Geometry check sheet. Reference: drawing and pictorial views, mm from the part's lowest x, y, z. A direction names the side the tool comes from. Coordinates: 2 decimals unless noted, no trailing zeros. Write each loop counter-clockwise with the first axis right and the second up, starting at its lowest first coordinate (ties: lowest second). Pieces come first, ordered by that corner, then holes. Notation, with made-up numbers: M -20.5,-10.75 L -2.5,-10.75 A19 cw -2.5,-0.75 Z; hole C 0,0 d2. An arc over 180 degrees is marked long. One line per item, written item: value.
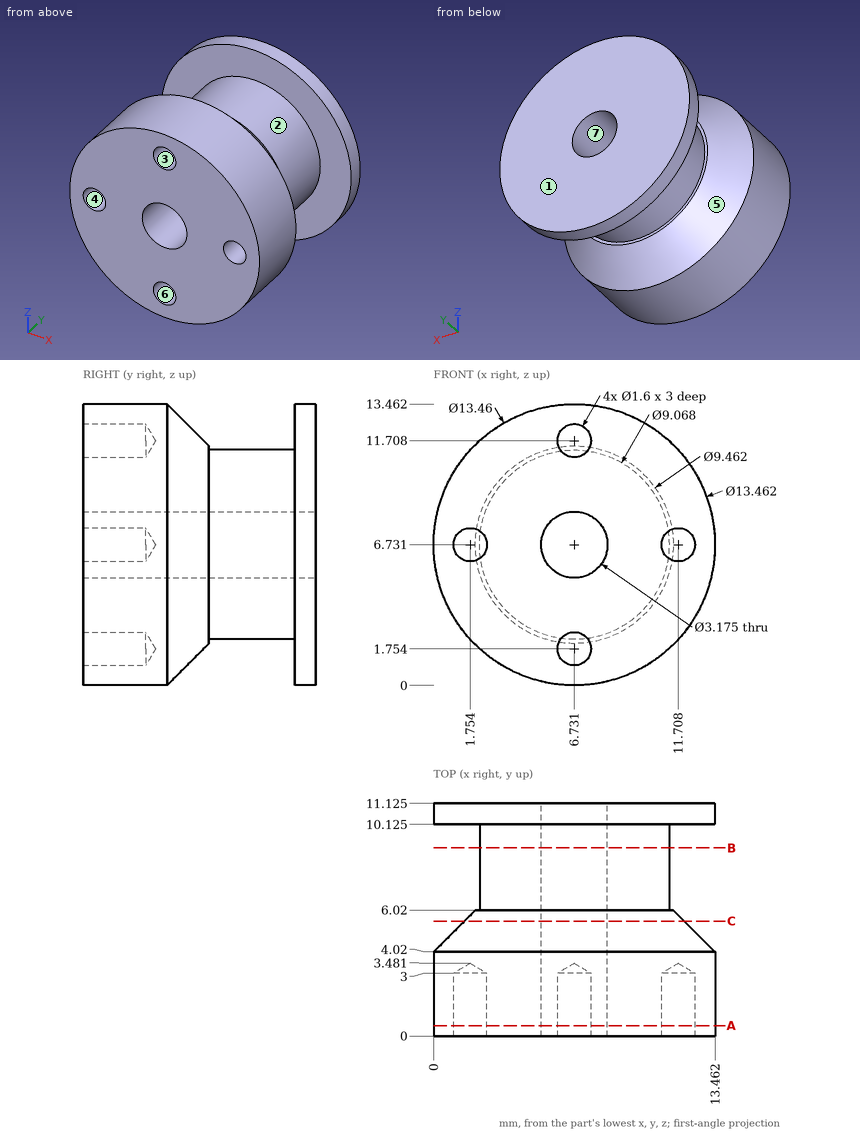
Item 1: Go/stop test with flat-tipped pins: P1, Ø6, axis at x = 11, y = 9.5, coming from the -Z side (1 decimal); P2, Ø1, axis at y = 4.5, z = 4, coming from the -X side; P3, Ø4, axis at y = 5.5, z = 11.5, coming from the +X side (1 decimal). Record where each tip stops, or that it passes through.
The answers:
P1: stops at z = 0.1
P2: stops at x = 0.52
P3: stops at x = 12.5
Item 2: Cross-section at B-B, the plane y = 9. Enter the section's corners in (x, z) (1 decimal).
The answers:
outline: C 6.7,6.7 d9.1; hole C 6.7,6.7 d3.2
Item 3: Cross-section at C-C, the plane y = 5.5. Enter the section's corners in (x, z) (1 decimal).
The answers:
outline: C 6.7,6.7 d10.5; hole C 6.7,6.7 d3.2
Item 4: Scan lines: line 1 (Y direction, x = 4.25, z = 10.75) (1 decimal); line 2 (Y direction, x = 13, z = 5.75) (1 decimal); line 3 (Z direction, x = 6.75, y = 5.25) (1 decimal). Record each from-to range of solid material in increasing order.
The answers:
line 1: y = 0 to 6, 10.1 to 11.1
line 2: y = 0 to 4.4, 10.1 to 11.1
line 3: z = 1.2 to 5.1, 8.3 to 12.2
Item 5: Cross-section at A-A, the plane y = 0.5. Enter the section's corners in (x, z) (1 decimal).
The answers:
outline: C 6.7,6.7 d13.5; hole C 1.8,6.7 d1.6; hole C 6.7,6.7 d3.2; hole C 6.7,1.8 d1.6; hole C 6.7,11.7 d1.6; hole C 11.7,6.7 d1.6
Item 6: Draft check along X on the marked faces 1, 2, 3 and 4. Enter one of: released by +X, released by -X, zero draft, split by the parting line, or undercut.
The answers:
face 1: zero draft
face 2: split by the parting line
face 3: undercut
face 4: undercut
Item 7: Access from +Z, -Z, +X, -X, +Y, -Y to the whole of each face (thin tool, end or side, straight path). Record for the marked faces 5, 6 and 7.
The answers:
face 5: none
face 6: -Y
face 7: +Y, -Y
